Input: dimensioned drawing with shaded views. Units: mm. Origin: part minimum x, y, z. A direction names the side the tool comes from. Round coordinates to 2 decimals unless told otherwise and drop trailing zeros. Order: outer loops, then holes, each group sorted by start corner. A loop starts at its lowest first (then second) coordinate and runs counter-clockwise, first axis right, second up. Notation, with made-up numbers: (28.5, 0) - (33.5, 0) arc R16 ccw to (33.5, 6) - close; hole circle Ø7 at (17, -40). An arc over 180 degrees is marked (long way). Return JSON: item names as keys, results as strings. Group by question number.
1) Section A-A, the plane z = 12.5. Return loops of the section in (x, y), plus the area to 3 significant figures.
2) Mould query, pull axis Z, two halves, no side actions, for the marked faces 1, 2 and 3. Classes: pulls with the +Z half, pulls with the -Z half, needs draft (parallel to the pull), parting line crosses it, or undercut.
3) Section B-B, the plane y = 3.5. Return loops of the section in (x, z), plus the area to 3 significant figures.
4) Section C-C, the plane z = 23. Return loops of the section in (x, y).
5) Ray query, line 1 (X direction, y = 4, z = 13.5); line 2 (X direction, y = 5, z = 22.25); line 3 (Z direction, x = 137.5, y = 5). Return the intervals inside material, ascending. Write a range as from..to.
6) Access query for the marked faces 4 and 5. Directions: +Z, -Z, +X, -X, +Y, -Y. A direction counts if a zero-diameter tool reaches every point of the face in a straight line with its end or side. Return the directions, or none.
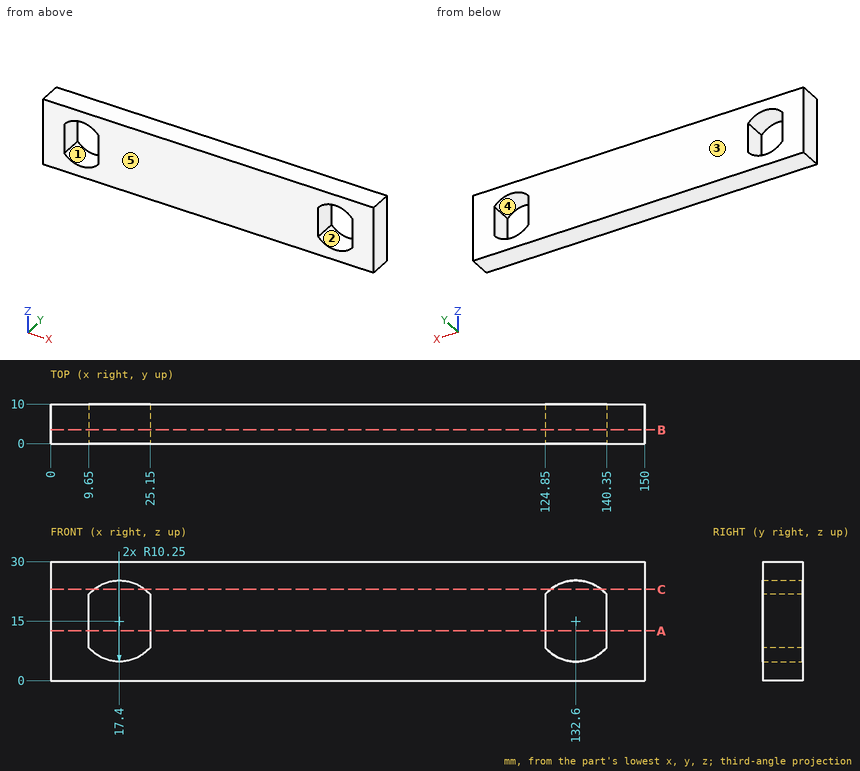
Geometry check:
{
 "1": {"outline": "(0, 0) - (9.65, 0) - (9.65, 10) - (0, 10) - close; (25.15, 0) - (124.85, 0) - (124.85, 10) - (25.15, 10) - close; (140.35, 0) - (150, 0) - (150, 10) - (140.35, 10) - close", "area": "1,190 mm2"},
 "2": {"face 1": "undercut", "face 2": "undercut", "face 3": "needs draft"},
 "3": {"outline": "(0, 0) - (150, 0) - (150, 30) - (0, 30) - close; hole (9.65, 8.29) arc R10.25 ccw to (25.15, 8.29) - (25.15, 21.71) arc R10.25 ccw to (9.65, 21.71) - close; hole (124.85, 8.29) arc R10.25 ccw to (140.35, 8.29) - (140.35, 21.71) arc R10.25 ccw to (124.85, 21.71) - close", "area": "3,930 mm2"},
 "4": {"outline": "(0, 0) - (10.99, 0) - (10.99, 10) - (0, 10) - close; (23.81, 0) - (126.19, 0) - (126.19, 10) - (23.81, 10) - close; (139.01, 0) - (150, 0) - (150, 10) - (139.01, 10) - close"},
 "5": {"line 1": "0..9.65, 25.15..124.85, 140.35..150", "line 2": "0..10.15, 24.65..125.35, 139.85..150", "line 3": "0..6, 24..30"},
 "6": {"face 4": "+Y, -Y", "face 5": "+Z, -Z, +X, -X, -Y"}
}
